Read the model definition and answer for the solid it produces. Units are mm, in the model's axes. A direction names the side the tool comes from. Coordinates: 2 decimals unless noted, no trailing zeros. Order: outer loops, then holes, each group sorted by start corner. A loop starts at its lowest first (then second) coordinate and runs counter-clockwise, first axis right, second up. Notation, with made-up numbers: (76.5, 9.5) - (117.5, 9.5) arc R12 cw to (117.5, 13.5) - close; hole circle Ø2 at (48, 39.5). An arc over 180 degrees is marked (long way). Write item = value, one per line.
from build123d import *

# Parameters (mm, degrees)
SKETCH1_R               = 2.25
BOSS_EXTRUDE1_DEPTH     = 6
SKETCH2_R               = 10
CUT_EXTRUDE1_DEPTH      = 1.2
CUT_EXTRUDE2_DEPTH      = 54.27936377
CUT_EXTRUDE2_DEPTH_BACK = 54.27936377


with BuildPart() as part:
    # Sketch1 → Boss-Extrude1 (new body)
    with BuildSketch(Plane(origin=(0, 0, 0), x_dir=(1, 0, 0), z_dir=(0, 1, 0))):
        Polygon((0, 4.970562748), (0, -4.970562748), (6.829437252, -11.8), (39.85294373, -11.8), (39.86294373, -11.81), (40.05294373, -12), (42.371856048, -14.318912318), (46.04881131, -10.641957056), (46.04881131, 10.641957056), (42.371856048, 14.318912318), (40.05294373, 12), (39.86294373, 11.81), (39.85294373, 11.8), (6.829437252, 11.8), align=None)
        with Locations(Location((12, 0, 0), (0, 0, 270))):
            Circle(SKETCH1_R, mode=Mode.SUBTRACT)
    extrude(amount=BOSS_EXTRUDE1_DEPTH)

    # Sketch2 → Cut-Extrude1 (cut)
    with BuildSketch(Plane.XZ):
        with Locations(Location((12, 0, 0), (0, 0, 270))):
            Circle(SKETCH2_R)
    extrude(amount=-CUT_EXTRUDE1_DEPTH, mode=Mode.SUBTRACT)

    # Sketch3 → Cut-Extrude2 (cut, two sides: drawn at the far end of the back side and taken through both)
    with BuildSketch(Plane(origin=(0, 0, -11.8), x_dir=(-1, 0, 0), z_dir=(0, 0, -1)).offset(-CUT_EXTRUDE2_DEPTH_BACK)):
        Polygon((-46.04881131, 6), (0, 6), (0, 4), (-20, 4), (-42.371856048, 4.781242428), (-46.04881131, 4.781242428), align=None)
    extrude(amount=CUT_EXTRUDE2_DEPTH + CUT_EXTRUDE2_DEPTH_BACK, mode=Mode.SUBTRACT)


solid = part.part
1) The part is cut by section A-A (y = 1.65). Determine the outline of the cut face in (x, z).
Returned:
outline = (0, -4.97) - (6.83, -11.8) - (39.85, -11.8) - (42.37, -14.32) - (46.05, -10.64) - (46.05, 10.64) - (42.37, 14.32) - (39.85, 11.8) - (6.83, 11.8) - (0, 4.97) - close; hole circle Ø4.5 at (12, 0)
2) For faces 1 (the face through (10, 4, -2)), 2 (the face through (14.4, 1.2, 0.1)), 3 (the face through (24, 2, -11.8)), determine the directions among +Z, -Z, +X, -X, +Y, -Y from which every point of the face is accessible in a straight line to the end or side of a thin tool.
Returned:
face_1 = +Z, -Z, -X, +Y
face_2 = -Y
face_3 = -Z, -X, +Y, -Y
3) The part is cut by section B-B (x = 12). Determine the outline of the cut face in (y, z), and give its area (3 significant figures).
Returned:
outline = (0, -11.8) - (4, -11.8) - (4, -2.25) - (1.2, -2.25) - (1.2, -10) - (0, -10) - close; (0, 10) - (1.2, 10) - (1.2, 2.25) - (4, 2.25) - (4, 11.8) - (0, 11.8) - close
area = 57.8 mm^2
4) Determine the mould class of faces 4 (the face through (2.24, 0.59, 2.17)), 5 (the face through (23, 2, 11.8)), 6 (the face through (44.24, 2.36, -12.45)) for opening direction Z: pulls with the +Z half, pulls with the -Z half, needs draft (parallel to the pull), parting line crosses it, or undercut.
Returned:
face_4 = undercut
face_5 = pulls with the +Z half
face_6 = pulls with the -Z half
5) Straight lines are drawn through the part: line 1 along Z through (x, y) = (12, 2.45); line 2 along X through (y, z) = (0.9, 0); line 3 along Z through (x, y) = (26.5, 1.2). For each, find the intervals that lie inside material, in ascending order. Write a range as from..to.
Returned:
line_1 = -11.8..-2.25, 2.25..11.8
line_2 = 0..2, 22..46.05
line_3 = -11.8..11.8
6) The part is cut by section C-C (z = 0). Determine the outline of the cut face in (x, y).
Returned:
outline = (0, 0) - (2, 0) - (2, 1.2) - (9.75, 1.2) - (9.75, 4) - (0, 4) - close; (14.25, 1.2) - (22, 1.2) - (22, 0) - (46.05, 0) - (46.05, 4.78) - (42.37, 4.78) - (20, 4) - (14.25, 4) - close
7) Flat-ended cylindrical pins translate along their axes: pin 1 Ø2 at (x, y) = (27, 4) entering from +Z; pin 2 Ø2.5 at (x, y) = (29.5, 1.5) entering from -Z; pin 3 Ø10 at (x, z) = (10, -1) entering from -Y. Find the tip coordinate at first contact, or state that the pin passes through.
Returned:
pin_1 = 11.8
pin_2 = -11.8
pin_3 = 1.2
8) The part is cut by section D-D (z = 8.25). Determine the outline of the cut face in (x, y).
Returned:
outline = (3.28, 0) - (6.35, 0) - (6.35, 1.2) - (17.65, 1.2) - (17.65, 0) - (46.05, 0) - (46.05, 4.78) - (42.37, 4.78) - (20, 4) - (3.28, 4) - close
